Geometry check sheet. Reference: drawing and pictorial views, mm from the part's lowest x, y, z. Round coordinates to 2 decimals unless told otherwise and drop trailing zeros. Write each loop counter-clockwise with the first axis right and the second up, starting at its lowest first coordinate (ties: lowest second). Pieces come first, ordered by that corner, then holes. Notation, with made-up numbers: M 81,-20 L 109,-20 A15 ccw 109,-1 Z; hole C 30,5 d3. An arc over 180 degrees is marked long. Put each result on its own line as item: value. Start each with the question number.
(1) Material ranges on probe 1 along X at (y, z) = (19, 37), recorded low to high.
(2) Gauge pin test, flat ends, axial feed: pin 1 (7 mm diameter, centred on y = 67, z = 54.5, fed in from +X); pin 2 (8 mm diameter, centred on y = 73, z = 27, fed in from -X); pin 3 (15 mm diameter, centred on x = 15.5, z = 29.5, fed in from -Y). Record the tip position at first contact, or that the pin passes through.
(3) Section check B-B on y = 70. Record the cut outline in (x, z), then the cut area to 3 significant figures.
(4) Section check A-A on z = 54. Record the cut outline in (x, y).
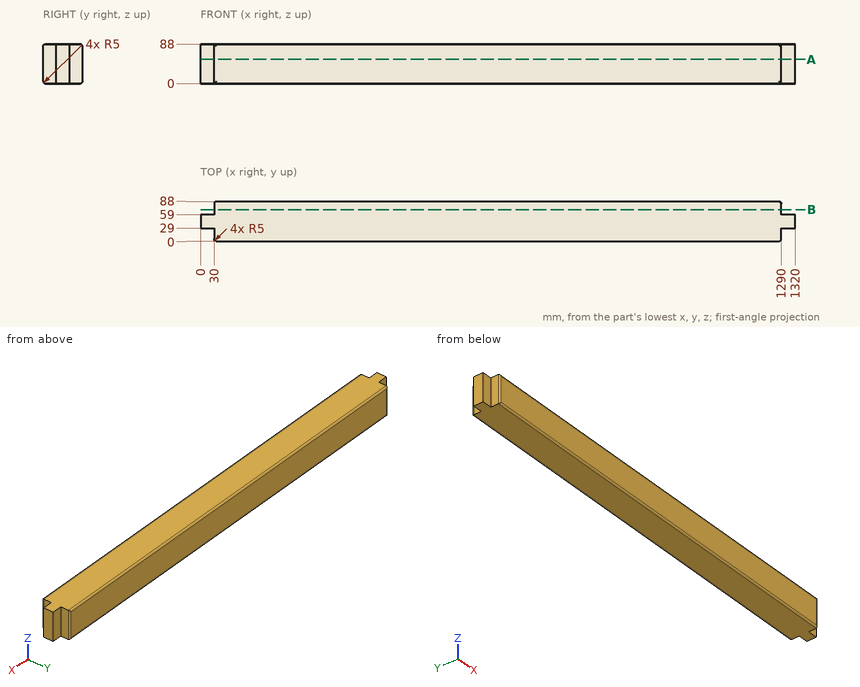
Answers follow:
1. probe 1: x = 30 to 1290
2. pin 1: stops at x = 1290
2. pin 2: stops at x = 30
2. pin 3: stops at y = 29
3. outline: M 30,0 L 1290,0 L 1290,88 L 30,88 Z
3. area: 111,000 mm^2
4. outline: M 0,29 L 30,29 L 30,5 A5 ccw 35,0 L 1285,0 A5 ccw 1290,5 L 1290,29 L 1320,29 L 1320,59 L 1290,59 L 1290,83 A5 ccw 1285,88 L 35,88 A5 ccw 30,83 L 30,59 L 0,59 Z
